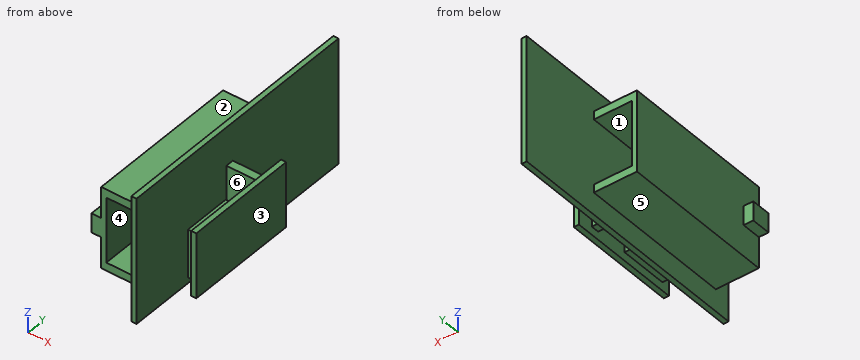
from build123d import *

# Parameters (mm, degrees)
EXTRUDE_1_DEPTH      = 0.8
EXTRUDE_1_DEPTH_BACK = 0.8
SKETCH_1_W           = 39.2
SKETCH_1_H           = 80
SKETCH_1_3_W         = 15.24
SKETCH_1_3_H         = 2.54
EXTRUDE_2_DEPTH      = 11.8
SKETCH_2_W           = 15.24
SKETCH_2_H           = 2.54
SKETCH_2_W_2         = 6
SKETCH_2_H_2         = 0.92
EXTRUDE_3_DEPTH      = 1.6
SKETCH_2_3_W         = 15
SKETCH_2_3_H         = 15
EXTRUDE_4_DEPTH      = 3
SKETCH_1_4_W         = 2.54
SKETCH_1_4_H         = 48.3
EXTRUDE_6_DEPTH      = 12.6
SKETCH_3_W           = 20.32
SKETCH_3_H           = 10.16
SKETCH_3_W_2         = 15.24
SKETCH_3_H_2         = 2.54
SKETCH_3_W_3         = 7.16
EXTRUDE_7_DEPTH      = 1.6
SKETCH_3_3_W         = 6
SKETCH_3_3_H         = 2.54
SKETCH_3_3_H_2       = 0.92
EXTRUDE_8_DEPTH      = 4.6


with BuildPart() as part:
    # Sketch 1 → Extrude 1 (new, two sides: drawn at the far end of the back side and taken through both)
    with BuildSketch(Plane(origin=(0, 0, 0), x_dir=(0, 0, -1), z_dir=(1, 0, 0)).offset(-EXTRUDE_1_DEPTH_BACK)):
        Rectangle(SKETCH_1_W, SKETCH_1_H)
    extrude(amount=EXTRUDE_1_DEPTH + EXTRUDE_1_DEPTH_BACK)

    # Sketch 1_3 → Extrude 2 (add)
    with BuildSketch(Plane(origin=(0, 0, 0), x_dir=(0, 0, -1), z_dir=(1, 0, 0))):
        with Locations((0, -3.13)):
            Rectangle(SKETCH_1_3_W, SKETCH_1_3_H)
    extrude(amount=EXTRUDE_2_DEPTH)

    # Sketch 2 → Extrude 3 (add)
    # profile 1 of 5: a face of its own
    with BuildSketch(Plane(origin=(11.8, 0, 0), x_dir=(0, 0, -1), z_dir=(1, 0, 0))):
        Polygon((-10.16, 3.22), (-10.16, -32.38), (-3, -32.38), (-3, -29.84), (-7.5, -29.84), (-7.5, -14.84), (7.5, -14.84), (7.5, -29.84), (3, -29.84), (3, -32.38), (10.16, -32.38), (10.16, 3.22), align=None)
        with Locations((0, -3.13)):
            Rectangle(SKETCH_2_W, SKETCH_2_H, mode=Mode.SUBTRACT)
    # profile 2 of 5: a face of its own
    with BuildSketch(Plane(origin=(11.8, 0, 0), x_dir=(0, 0, -1), z_dir=(1, 0, 0))):
        with Locations((0, -31.11)):
            Rectangle(SKETCH_2_W_2, SKETCH_2_H)
    # profile 3 of 5: a face of its own
    with BuildSketch(Plane(origin=(11.8, 0, 0), x_dir=(0, 0, -1), z_dir=(1, 0, 0))):
        with Locations((0, -3.13)):
            Rectangle(SKETCH_2_W, SKETCH_2_H)
    # profile 4 of 5: a face of its own
    with BuildSketch(Plane(origin=(11.8, 0, 0), x_dir=(0, 0, -1), z_dir=(1, 0, 0))):
        Polygon((-7.5, -29.84), (-3, -29.84), (-3, -28.92), (3, -28.92), (3, -29.84), (7.5, -29.84), (7.5, -14.84), (-7.5, -14.84), align=None)
    # profile 5 of 5: a face of its own
    with BuildSketch(Plane(origin=(11.8, 0, 0), x_dir=(0, 0, -1), z_dir=(1, 0, 0))):
        with Locations((0, -29.38)):
            Rectangle(SKETCH_2_W_2, SKETCH_2_H_2)
    extrude(amount=EXTRUDE_3_DEPTH)

    # Sketch 2_3 → Extrude 4 (add)
    with BuildSketch(Plane(origin=(11.8, 0, 0), x_dir=(0, 0, -1), z_dir=(1, 0, 0))):
        with Locations((0, -22.34)):
            Rectangle(SKETCH_2_3_W, SKETCH_2_3_H)
    extrude(amount=-EXTRUDE_4_DEPTH)

    # Sketch 1_4 → Extrude 6 (add)
    with BuildSketch(Plane(origin=(0, 0, 0), x_dir=(0, 0, -1), z_dir=(1, 0, 0))):
        with Locations((-11.43, -10.77)):
            Rectangle(SKETCH_1_4_W, SKETCH_1_4_H)
        with Locations((11.43, -10.77)):
            Rectangle(SKETCH_1_4_W, SKETCH_1_4_H)
    extrude(amount=-EXTRUDE_6_DEPTH)

    # Sketch 3 → Extrude 7 (add)
    # profile 1 of 8: a face of its own
    with BuildSketch(Plane.ZY.offset(12.6)):
        Polygon((-10.16, 3.22), (-10.16, 13.38), (-12.7, 13.38), (-12.7, -34.92), (-10.16, -34.92), (-10.16, -32.38), align=None)
    # profile 2 of 8: a face of its own
    with BuildSketch(Plane.ZY.offset(12.6)):
        with Locations((0, 8.3)):
            Rectangle(SKETCH_3_W, SKETCH_3_H)
    # profile 3 of 8: a face of its own
    with BuildSketch(Plane.ZY.offset(12.6)):
        Polygon((12.7, 13.38), (10.16, 13.38), (10.16, 3.22), (10.16, -32.38), (10.16, -34.92), (12.7, -34.92), align=None)
    # profile 4 of 8: a face of its own
    with BuildSketch(Plane.ZY.offset(12.6)):
        Polygon((10.16, 3.22), (-10.16, 3.22), (-10.16, -32.38), (-3, -32.38), (-3, -29.84), (-7.5, -29.84), (-7.5, -14.84), (7.5, -14.84), (7.5, -29.84), (3, -29.84), (3, -32.38), (10.16, -32.38), align=None)
        with Locations((0, -3.13)):
            Rectangle(SKETCH_3_W_2, SKETCH_3_H_2, mode=Mode.SUBTRACT)
    # profile 5 of 8: a face of its own
    with BuildSketch(Plane.ZY.offset(12.6)):
        with Locations((0, -3.13)):
            Rectangle(SKETCH_3_W_2, SKETCH_3_H_2)
    # profile 6 of 8: a face of its own
    with BuildSketch(Plane.ZY.offset(12.6)):
        Polygon((-7.5, -29.84), (-3, -29.84), (-3, -28.92), (3, -28.92), (3, -29.84), (7.5, -29.84), (7.5, -14.84), (-7.5, -14.84), align=None)
    # profile 7 of 8: a face of its own
    with BuildSketch(Plane.ZY.offset(12.6)):
        with Locations((-6.58, -33.65)):
            Rectangle(SKETCH_3_W_3, SKETCH_3_H_2)
    # profile 8 of 8: a face of its own
    with BuildSketch(Plane.ZY.offset(12.6)):
        with Locations((6.58, -33.65)):
            Rectangle(SKETCH_3_W_3, SKETCH_3_H_2)
    extrude(amount=EXTRUDE_7_DEPTH)

    # Sketch 3_3 → Extrude 8 (add)
    with BuildSketch(Plane.ZY.offset(12.6)):
        with Locations((0, -33.65)):
            Rectangle(SKETCH_3_3_W, SKETCH_3_3_H)
        with Locations((0, -31.11)):
            Rectangle(SKETCH_3_3_W, SKETCH_3_3_H)
        with Locations((0, -29.38)):
            Rectangle(SKETCH_3_3_W, SKETCH_3_3_H_2)
    extrude(amount=EXTRUDE_8_DEPTH)


solid = part.part
Verification items for the finished model (mm, model axes). Face numbers are marked on the shaded views. A direction names the side the tool comes from. Coordinates: 2 decimals unless noted, no trailing zeros. Order: outer loops, then holes, each group sorted by start corner. A loop starts at its lowest first (then second) coordinate and runs counter-clockwise, first axis right, second up. Notation, with made-up numbers: M 3,46.25 L 23,46.25 A35 ccw 23,85.25 Z; hole C 67,36.5 d2. An arc over 180 degrees is marked long. One line per item, written item: value. Start each with the question number.
Item 1: Sectioned sample at A-A on y = -26. Record the cut outline in (x, z), then the cut area to 3 significant figures.
Item 2: Mould release check, pull along X, two halves, no side actions. Record for the marked faces 1, 2 and 3: pulls with the +X half, pulls with the -X half, needs draft (parallel to the pull), parting line crosses it, or undercut.
Item 3: Sectioned sample at B-B on x = -7. Record the cut outline in (y, z).
Item 4: Access from +Z, -Z, +X, -X, +Y, -Y to the whole of each face (thin tool, end or side, straight path). Record for the marked faces 4, 5 and 6.
Item 5: Depth check by flat-ended pin: P1, Ø4.5, axis at y = -22.5, z = -1.5, coming from the -X side; P2, Ø1.8, axis at x = 12.5, y = -15, coming from the -Z side; P3, Ø1.8, axis at x = 12, z = -0.5, coming from the +Y side. Enter the tip coordinate at first touch or a pass-through.
Item 6: Sectioned sample at D-D on y = -0.5. Record the cut outline in (x, z), then the cut area to 3 significant figures.
Item 7: Thickness scan on probe 1 along X at (y, z) = (-25.5, -1.5); probe 2 along X at (y, z) = (7.5, 1); probe 3 along Z at (x, y) = (-6, 2). Record the ranges inside material, lowest first.
Item 8: Sectioned sample at C-C on z = -6. Record the cut outline in (x, y).
Calculated:
1. outline: M -14.2,-12.7 L -0.8,-12.7 L -0.8,-19.6 L 0.8,-19.6 L 0.8,19.6 L -0.8,19.6 L -0.8,12.7 L -14.2,12.7 Z; M 8.8,-7.5 L 11.8,-7.5 L 11.8,-10.16 L 13.4,-10.16 L 13.4,10.16 L 11.8,10.16 L 11.8,7.5 L 8.8,7.5 Z; hole M -12.6,-10.16 L -0.8,-10.16 L -0.8,10.16 L -12.6,10.16 Z
1. area: 241 mm^2
2. face 1: undercut
2. face 2: needs draft
2. face 3: pulls with the +X half
3. outline: M -34.92,-12.7 L 13.38,-12.7 L 13.38,-10.16 L -34.92,-10.16 Z; M -34.92,10.16 L 13.38,10.16 L 13.38,12.7 L -34.92,12.7 Z
4. face 4: +Y, -Y
4. face 5: -Z, -X, +Y, -Y
4. face 6: +Z, -Z
5. P1: x = -14.2
5. P2: z = -10.16
5. P3: y = 3.22
6. outline: M -14.2,-12.7 L -0.8,-12.7 L -0.8,-19.6 L 0.8,-19.6 L 0.8,19.6 L -0.8,19.6 L -0.8,12.7 L -14.2,12.7 Z; M 11.8,-10.16 L 13.4,-10.16 L 13.4,10.16 L 11.8,10.16 Z; hole M -12.6,-10.16 L -0.8,-10.16 L -0.8,10.16 L -12.6,10.16 Z
6. area: 196 mm^2
7. probe 1: -14.2 to -12.6, -0.8 to 0.8, 8.8 to 13.4
7. probe 2: -14.2 to -12.6, -0.8 to 0.8
7. probe 3: -12.7 to -10.16, 10.16 to 12.7
8. outline: M -14.2,-34.92 L -12.6,-34.92 L -12.6,13.38 L -14.2,13.38 Z; M -0.8,-40 L 0.8,-40 L 0.8,-4.4 L 11.8,-4.4 L 11.8,-14.84 L 8.8,-14.84 L 8.8,-29.84 L 11.8,-29.84 L 11.8,-32.38 L 13.4,-32.38 L 13.4,3.22 L 11.8,3.22 L 11.8,-1.86 L 0.8,-1.86 L 0.8,40 L -0.8,40 Z
